```python
from build123d import *

# Parameters (mm, degrees)
BOX085084_W                                                = 8.1
BOX085084_H                                                = 10
BOX085084_DEPTH                                            = 15.8
FILLET005011017044_R                                       = 3.25
CYLINDER053_R                                              = 1.6
CYLINDER053_DEPTH                                          = 10
CYLINDER054_R                                              = 1.6
CYLINDER054_DEPTH                                          = 10
FUSION004008002002002001007002002026012008_PLACEMENT_ANGLE = 90
BOX085130_W                                                = 29.5
BOX085130_H                                                = 1
BOX085130_DEPTH                                            = 14.5
CHAMFER011006003017049_SIZE                                = 0.98


with BuildPart() as fillet005011017044:
    # Box085084 → Box085084 (new body)
    with BuildSketch(Plane(origin=(15.9, 118, 17.9), x_dir=(1, 0, 0), z_dir=(0, 0, 1))):
        with Locations((4.05, 5)):
            Rectangle(BOX085084_W, BOX085084_H)
    extrude(amount=BOX085084_DEPTH)

    # Fillet005011017044
    fillet005011017044_edges = [fillet005011017044.edges().sort_by_distance(p)[0] for p in [
        (15.9, 123, 33.7),
        (24, 123, 33.7),
    ]]
    fillet(fillet005011017044_edges, radius=FILLET005011017044_R)


with BuildPart() as cylinder053:
    # Cylinder053 → Cylinder053 (new body)
    with BuildSketch(Plane(origin=(20, 128, 15.5), x_dir=(1, 0, 0), z_dir=(0, -1, 0))):
        Circle(CYLINDER053_R)
    extrude(amount=CYLINDER053_DEPTH)


with BuildPart() as obj1:
    # Cylinder054 → Cylinder054 (new body)
    with BuildSketch(Plane(origin=(20, 128, 36.1), x_dir=(1, 0, 0), z_dir=(0, -1, 0))):
        Circle(CYLINDER054_R)
    extrude(amount=CYLINDER054_DEPTH)

    # Fusion004008002002002001007002002026012008: union Fillet005011017044, Cylinder053
    add(fillet005011017044.part)
    add(cylinder053.part)


with BuildPart() as obj1_1:
    # Fusion004008002002002001007002002026012008 placement: moved
    add(obj1.part.moved(Location((149.7, -4, 13.1))).rotate(Axis((149.7, -4, 13.1), (0, -1, 0)), FUSION004008002002002001007002002026012008_PLACEMENT_ANGLE))


with BuildPart() as cut001002016041:
    # Box085130 → Box085130 (new body)
    with BuildSketch(Plane(origin=(113.15, 117, 27.8), x_dir=(1, 0, 0), z_dir=(0, 0, 1))):
        with Locations((14.75, 0.5)):
            Rectangle(BOX085130_W, BOX085130_H)
    extrude(amount=BOX085130_DEPTH)

    # Chamfer011006003017049
    chamfer011006003017049_edges = [cut001002016041.edges().sort_by_distance(p)[0] for p in [
        (113.15, 117, 35.05),
        (142.65, 117, 35.05),
        (127.9, 117, 27.8),
        (127.9, 117, 42.3),
    ]]
    chamfer(chamfer011006003017049_edges, length=CHAMFER011006003017049_SIZE)


with BuildPart() as cut001002016041_1:
    # Chamfer011006003017049 placement: moved
    add(cut001002016041.part.moved(Location((-4, 0, -2))))

    # Cut001002016041: cut obj1
    add(obj1_1.part, mode=Mode.SUBTRACT)


solid = cut001002016041_1.part
```
Check sheet for the modelled part. Datum: model origin and axes. Units: mm. A direction names the side the tool comes from. Round coordinates to 2 decimals unless told otherwise and drop trailing zeros. Loops run counter-clockwise (first coordinate to the right, second up) from the corner with the lowest first, then second, coordinate; pieces in that order, holes last. Notation, with made-up numbers: (42, -26.5) - (62, -26.5) arc R26 ccw to (62, 5.5) - close; hole circle Ø7 at (3, -33.5). An arc over 180 degrees is marked (long way). Write item = value, one per line. Start each with the question number.
Q1. Depth check by flat-ended pin: P1, Ø3, axis at x = 122.5, z = 31.5, coming from the -Y side; P2, Ø0.5, axis at y = 117.5, z = 31.5, coming from the -X side; P3, Ø0.5, axis at x = 126, y = 117.5, coming from the +Z side; P4, Ø0.5, axis at y = 117.5, z = 33, coming from the +X side. Enter the tip coordinate at first touch or a pass-through.
Q2. Section check B-B (z = 33.1). Count the separate pieces of the cut face and the enclosed holes in it, plus the area to 3 significant figures.
Q3. Thickness scan on L1, parallel to X at y = 117.35, z = 33.1; L2, parallel to X at y = 117.4, z = 33.1; L3, parallel to X at y = 117.3, z = 35.5. Record the ranges inside material, lowest first.
Q4. Section check C-C (y = 117.4). Record the boundary of the cut face in (x, z), plus the area to 3 significant figures.
Q5. Release check for a two-part mould opening along X. For faces 1 (the face through (123.69, 117.5, 26.28)), 2 (the face through (135.76, 117.51, 32.75)), 3 (the face through (138.17, 117.5, 32.95)) record: pulls with the +X half, pulls with the -X half, needs draft (parallel to the pull), parting line crosses it, or undercut.
Q6. Access from +Z, -Z, +X, -X, +Y, -Y to the whole of each face (thin tool, end or side, straight path). Record for faces 4 (the face through (109.65, 117.48, 32.95)), 5 (the face through (125.6, 117.5, 29)).
Derived:
q1.P1 = through
q1.P2 = 109.38
q1.P3 = 40.07
q1.P4 = 138.42
q2.separate_pieces = 4
q2.enclosed_holes = 0
q2.area = 6.34 mm^2
q3.L1 = 109.78 to 112, 115.2 to 116, 131.8 to 132.6, 135.8 to 138.02
q3.L2 = 109.73 to 112, 115.2 to 116, 131.8 to 132.6, 135.8 to 138.07
q3.L3 = 109.83 to 116.45, 131.8 to 137.97
q4.outline = (109.73, 26.38) - (138.07, 26.38) - (138.07, 39.72) - (109.73, 39.72) - close; hole circle Ø3.2 at (113.6, 33.1); hole (116, 32.25) arc R3.25 ccw to (119.25, 29) - (131.8, 29) - (131.8, 37.1) - (119.25, 37.1) arc R3.25 ccw to (116, 33.85) - close; hole circle Ø3.2 at (134.2, 33.1)
q4.area = 239 mm^2
q5.face_1 = needs draft
q5.face_2 = undercut
q5.face_3 = pulls with the +X half
q6.face_4 = +Z, -Z, -X, -Y
q6.face_5 = +Y, -Y
